```python
from build123d import *

# Parameters (mm, degrees)
SKETCH2_RX          = 47.005912867
SKETCH2_RY          = 10.001258057
BOSS_EXTRUDE2_DEPTH = 29
BOSS_EXTRUDE3_DEPTH = 4
BOSS_EXTRUDE4_DEPTH = 70


with BuildPart() as part:
    # Sketch2 → Boss-Extrude2 (new body)
    with BuildSketch(Plane.XY):
        with Locations(Location((-67.802373164, 6.5712636), (0, 0, 0.908793004))):
            Ellipse(SKETCH2_RX, SKETCH2_RY)
    extrude(amount=BOSS_EXTRUDE2_DEPTH)

    # Sketch3 → Boss-Extrude3 (add)
    with BuildSketch(Plane(origin=(0, 0, 0), x_dir=(1, 0, 0), z_dir=(0, 1, 0))):
        with BuildLine():
            Line((-96.108391235, -29), (-39.496355092, -29))
            ThreePointArc((-39.496355092, -29), (-35.998589441, -14.5), (-39.496355092, 0))
            Line((-39.496355092, 0), (-96.108391235, 0))
            ThreePointArc((-96.108391235, 0), (-99.606156886, -14.5), (-96.108391235, -29))
        make_face()
    extrude(amount=-BOSS_EXTRUDE3_DEPTH)

    # Sketch5 → Boss-Extrude4 (add)
    with BuildSketch(Plane(origin=(0, 7.999999876, 0), x_dir=(-1, 0, 0), z_dir=(0, -1, 0))):
        with BuildLine():
            Line((44.932105476, 5.499725114), (90.672640852, 5.499725114))
            ThreePointArc((90.672640852, 5.499725114), (96.172365966, 0), (90.672640852, -5.499725114))
            Line((90.672640852, -5.499725114), (44.932105476, -5.499725114))
            ThreePointArc((44.932105476, -5.499725114), (39.432380362, 0), (44.932105476, 5.499725114))
        make_face()
    extrude(amount=-BOSS_EXTRUDE4_DEPTH)


solid = part.part
```
Here's how the part is built. I have some questions about the finished solid (model axes, mm). A direction names the side the tool comes from. Give positions to 0.01 mm unless a question says otherwise; leave off trailing zeros. Order: outer loops, then holes, each group sorted by start corner. A loop starts at its lowest first (then second) coordinate and runs counter-clockwise, first axis right, second up. Notation, with made-up numbers: (28.25, 28.25) - (66.25, 28.25) arc R17 ccw to (66.25, 52.25) - close; hole circle Ø4 at (5.5, 1.5). An arc over 180 degrees is marked (long way). Answer as a JSON object with one key per item and string values. Group by question number.
Item 1: Please list where these lines run through material, in increasing order: probe 1 along Z at (x, y) = (-50.5, 48); probe 2 along Z at (x, y) = (-75.5, 3.5); probe 3 along X at (y, z) = (48.5, 0).
Item 2: If we mould it in two halves opening along Y, with no side actions, what happens to faces 1 (the cylindrical face through (-96.17, 42.51, -0.12)), 2 (the flat face through (-68, 78, 0)), 3 (the flat face through (-68, 8, -3))? For each: pulls with the +Y half, pulls with the -Y half, needs draft (parallel to the pull), parting line crosses it, or undercut.
Item 3: For P1, Ø2, axis at x = -97.5, y = 55.5, coming from the -Z side; P2, Ø12, axis at x = -36, y = 20.5, coming from the -Z side; P3, Ø2, axis at x = -64.5, z = 20.5, coming from the +Y side; P4, Ø3, axis at y = 34.5, z = 3.5, coming from the +X side, each with a flat end and sliding along its axis, tell me the tip position at first contact or that it passes through.
Item 4: Which directions (+Z, -Z, +X, -X, +Y, -Y) give clear straight access to the entire face, cutting with the end or side of a thin tool? Please do faces 4 (the cylindrical face through (-36, -2.1, 14.7)), 5 (the flat face through (-68, 6, 29)), 6 (the cylindrical face through (-99.605, -2.618, 14.289)), 7 (the cylindrical face through (-39.434, 42.51, 0.121)).
Item 5: If we section it at A-A on y = 52: Please give me the cut outline in (x, z).
Result set:
{
 "1": {"probe 1": "-5.5 to 5.5", "probe 2": "0 to 29", "probe 3": "-96.17 to -39.43"},
 "2": {"face 1": "needs draft", "face 2": "pulls with the +Y half", "face 3": "pulls with the -Y half"},
 "3": {"P1": "through", "P2": "z = -4.65", "P3": "y = 16.6", "P4": "x = -39.81"},
 "4": {"face 4": "+X, -Y", "face 5": "+Z, +X, -X, +Y, -Y", "face 6": "-X, -Y", "face 7": "+X, +Y"},
 "5": {"outline": "(-90.67, -5.5) - (-44.93, -5.5) arc R5.5 ccw to (-44.93, 5.5) - (-90.67, 5.5) arc R5.5 ccw to start"}
}
